Check sheet for the modelled part. Datum: model origin and axes. Units: mm. A direction names the side the tool comes from. Give positions to 0.01 mm unless a question says otherwise; leave off trailing zeros. Loops run counter-clockwise (first coordinate to the right, second up) from the corner with the lowest first, then second, coordinate; pieces in that order, holes last. Notation, with made-up numbers: M 86,72.25 L 141,72.25 A16 cw 141,86.25 Z; hole C -29,-28 d7. An arc over 180 degrees is marked long. Use one line per item in the form item = value.
from build123d import *

# Parameters (mm, degrees)
F1_DEPTH = 25.4
F3_DEPTH = 25.401


with BuildPart() as f1:
    # F0 (on Front) → F1 (new body)
    with BuildSketch(Plane.XZ):
        with BuildLine():
            Line((584.2, 152.4), (-584.2, 152.4))
            Line((-584.2, 152.4), (-584.2, -152.4))
            ThreePointArc((-584.2, -152.4), (0, -240.490442), (584.2, -152.4))
            Line((584.2, -152.4), (584.2, 152.4))
        make_face()
    extrude(amount=F1_DEPTH)

    # F2 (on face) → F3 (cut, through all)
    with BuildSketch(Plane.XZ.offset(25.4)):
        with BuildLine():
            Line((558.8, -133.56262), (558.8, 152.4))
            Line((558.8, 152.4), (-558.8, 152.4))
            Line((-558.8, 152.4), (-558.8, -133.56262))
            ThreePointArc((-558.8, -133.56262), (0, -215.090442), (558.8, -133.56262))
        make_face()
    extrude(amount=-F3_DEPTH, mode=Mode.SUBTRACT)


solid = f1.part
1) Release check for a two-part mould opening along X. For faces 3 (the face through (572, -13, 152.4)), 4 (the face through (558.8, -13, 7)), 5 (the face through (-584.2, -13, 2)) record: pulls with the +X half, pulls with the -X half, needs draft (parallel to the pull), parting line crosses it, or undercut.
Evaluation:
face_3 = needs draft
face_4 = undercut
face_5 = pulls with the -X half
2) Scan lines: line 1 (X direction, y = -13, z = -130); line 2 (Z direction, x = 533, y = -21); line 3 (Z direction, x = 472, y = -20.75). Record each from-to range of solid material in increasing order.
Evaluation:
line_1 = -584.2 to -558.8, 558.8 to 584.2
line_2 = -167.45 to -141.06
line_3 = -183.44 to -157.28
3) Section check B-B (y = -17). Record the cut outline in (x, z), then the cut area to 3 significant figures.
Evaluation:
outline = M -584.2,-152.4 A1981.2 ccw 584.2,-152.4 L 584.2,152.4 L 558.8,152.4 L 558.8,-133.56 A1955.8 cw -558.8,-133.56 L -558.8,152.4 L -584.2,152.4 Z
area = 44,500 mm^2
4) Section check A-A (z = 88). Record the cut outline in (x, y).
Evaluation:
outline = M -584.2,-25.4 L -558.8,-25.4 L -558.8,0 L -584.2,0 Z; M 558.8,-25.4 L 584.2,-25.4 L 584.2,0 L 558.8,0 Z
5) Section check D-D (x = -264). Record the cut outline in (y, z).
Evaluation:
outline = M -25.4,-222.82 L 0,-222.82 L 0,-197.19 L -25.4,-197.19 Z
6) Set-up check for faces 1 (the face through (-558.8, -13, 11)), 2 (the face through (-8.302, -12.522, -240.473)): record each of +Z, -Z, +X, -X, +Y, -Y from which the full face is reachable in a straight line by a thin tool's end or side.
Evaluation:
face_1 = +Z, +Y, -Y
face_2 = -Z, +Y, -Y
7) Depth check by flat-ended pin: pin 1 Ø5 at (x, y) = (223, -10.5) entering from +Z. Enter the tip coordinate at first touch or a pass-through.
Evaluation:
pin_1 = -202.05
